Source: CAD feature listing. Evaluate the final solid. Frame: model axes, mm. A direction names the side the tool comes from. Round coordinates to 2 decimals unless told otherwise and drop trailing zeros. Loops run counter-clockwise (first coordinate to the right, second up) from the corner with the lowest first, then second, coordinate; pieces in that order, holes last. Notation, with made-up numbers: (-27, 35.25) - (8, 35.25) arc R22 cw to (8, 45.25) - close; hole circle Ø9 at (-27, -5). An arc over 180 degrees is marked (long way). One line per question, with ' | ' between items. Start each with the question number.
1. Cut plane D-D (x = 8). Return loops of the section in (y, z).
2. Pin query (flat end, axial travel): pin 1 (2 mm diameter, centred on x = 18, y = 0, fed in from -Z); pin 2 (1 mm diameter, centred on x = 7, z = 1.5, fed in from +Y). Return the tip coordinate at first contact, or that it passes through.
3. Ray query, line 1 (Y direction, x = -24, z = 0.45); line 2 (X direction, y = 1.25, z = 0.3); line 3 (Y direction, x = -30, z = 1.5). Return the intervals inside material, ascending.
4. Mould query, pull axis X, two halves, no side actions, for faces 1 (the flat face through (0, 0, 2)), 2 (the cylindrical face through (18.86, 0.27, 0.99)). Classes: pulls with the +X half, pulls with the -X half, needs draft (parallel to the pull), parting line crosses it, or undercut.
5. Access query for faces 3 (the cylindrical face through (-26, 0, 1)), 4 (the cylindrical face through (19.509, 3.287, 0.986)), 5 (the cylindrical face through (19.46, -3.27, 0.99)). Directions: +Z, -Z, +X, -X, +Y, -Y. A direction counts if a zero-diameter tool reaches every point of the face in a straight line with its end or side. Return the directions, or none.
6. Cut plane B-B (z = 0.35). State how many separate pieces and enclosed holes the cut face has, then the cut area to 3 significant figures.
7. Cut plane A-A (x = -12). Return loops of the section in (y, z).
8. Cut plane C-C (x = -24). Return loops of the section in (y, z).
```python
from build123d import *

# Parameters (mm, degrees)
F0_R     = 0.9
F0_R_2   = 2
F1_DEPTH = 2


with BuildPart() as f1:
    # F0 (on Top) → F1 (new body)
    with BuildSketch(Plane.XY):
        with BuildLine():
            Line((-17.6754446797, -3), (0, -3))
            Line((0, -3), (17.6754446797, -3))
            ThreePointArc((17.6754446797, -3), (19.4845127471, -3.2792244645), (21.1252021271, -4.0909090909))
            ThreePointArc((21.1252021271, -4.0909090909), (24.3345748945, -4.9887934052), (27.3953125, -3.6704022978))
            ThreePointArc((27.3953125, -3.6704022978), (28.474361287, -3.0297630587), (29.721059322, -2.8865536715))
            ThreePointArc((29.721059322, -2.8865536715), (32.9, 0), (29.721059322, 2.8865536715))
            ThreePointArc((29.721059322, 2.8865536715), (28.474361287, 3.0297630587), (27.3953125, 3.6704022978))
            ThreePointArc((27.3953125, 3.6704022978), (24.3345748945, 4.9887934052), (21.1252021271, 4.0909090909))
            ThreePointArc((21.1252021271, 4.0909090909), (19.4845127471, 3.2792244645), (17.6754446797, 3))
            Line((17.6754446797, 3), (0, 3))
            Line((0, 3), (-17.6754446797, 3))
            ThreePointArc((-17.6754446797, 3), (-19.4845127471, 3.2792244645), (-21.1252021271, 4.0909090909))
            ThreePointArc((-21.1252021271, 4.0909090909), (-24.3345748945, 4.9887934052), (-27.3953125, 3.6704022978))
            ThreePointArc((-27.3953125, 3.6704022978), (-28.474361287, 3.0297630587), (-29.721059322, 2.8865536715))
            ThreePointArc((-29.721059322, 2.8865536715), (-32.9, 0), (-29.721059322, -2.8865536715))
            ThreePointArc((-29.721059322, -2.8865536715), (-28.474361287, -3.0297630587), (-27.3953125, -3.6704022978))
            ThreePointArc((-27.3953125, -3.6704022978), (-24.3345748945, -4.9887934052), (-21.1252021271, -4.0909090909))
            ThreePointArc((-21.1252021271, -4.0909090909), (-19.4845127471, -3.2792244645), (-17.6754446797, -3))
        make_face()
        with Locations((-30, 0)):
            Circle(F0_R, mode=Mode.SUBTRACT)
        with Locations((-24, 0)):
            Circle(F0_R_2, mode=Mode.SUBTRACT)
        with Locations((-18, 0)):
            Circle(F0_R, mode=Mode.SUBTRACT)
        with Locations((-12, 0)):
            Circle(F0_R, mode=Mode.SUBTRACT)
        with Locations((12, 0)):
            Circle(F0_R, mode=Mode.SUBTRACT)
        with Locations((18, 0)):
            Circle(F0_R, mode=Mode.SUBTRACT)
        with Locations((24, 0)):
            Circle(F0_R_2, mode=Mode.SUBTRACT)
        with Locations((30, 0)):
            Circle(F0_R, mode=Mode.SUBTRACT)
    extrude(amount=F1_DEPTH)


solid = f1.part
```
Answers follow:
1) outline: (-3, 0) - (3, 0) - (3, 2) - (-3, 2) - close
2) pin 1: stops at z = 0 | pin 2: stops at y = 3
3) line 1: y = -5 to -2, 2 to 5 | line 2: x = -32.62 to -25.56, -22.44 to 22.44, 25.56 to 32.62 | line 3: y = -2.9 to -0.9, 0.9 to 2.9
4) face 1: needs draft | face 2: undercut
5) face 3: +Z, -Z | face 4: +Z, -Z, +Y | face 5: +Z, -Z, -Y
6) separate pieces: 1 | enclosed holes: 8 | area: 393 mm2
7) outline: (-3, 0) - (-0.9, 0) - (-0.9, 2) - (-3, 2) - close; (0.9, 0) - (3, 0) - (3, 2) - (0.9, 2) - close
8) outline: (-5, 0) - (-2, 0) - (-2, 2) - (-5, 2) - close; (2, 0) - (5, 0) - (5, 2) - (2, 2) - close
